CAD build for the part. Positions are in the model's coordinates, mm. A direction names the side the tool comes from. Round coordinates to 2 decimals unless told otherwise and drop trailing zeros. Loops run counter-clockwise (first coordinate to the right, second up) from the corner with the lowest first, then second, coordinate; pieces in that order, holes last. Notation, with made-up numbers: M -0.75,54 L 43.25,54 A19 cw 43.25,87 Z; hole C 35,21.25 d11. An arc over 180 degrees is marked long. Use a Markdown table: item, result. Add a question column.
(1) Band-saw the part on B-B, the plane y = 12. Write the cut outline in (x, z).
(2) Which spindle directions (+Z, -Z, +X, -X, +Y, -Y) get a long thin tool onto all of the face, cutting with end or side? Do faces 4 (the face through (124.456, 4, 13)), 5 (the face through (-81, 27, 25.4)). Say none if no direction does.
(3) Flat gauge pins, fed straight in: P1, Ø2, axis at x = 95.5, y = -0.5, coming from the +Z side; P2, Ø1, axis at x = -89.5, z = 43.5, coming from the +Y side; P3, Ø8, axis at y = 27.5, z = 36.5, coming from the -X side. Where does each tip first touch, or does it go through?
(4) Wall check: L1, parallel to Z at x = 68, y = -40.5; L2, parallel to X at y = 32, z = 48; L3, parallel to X at y = 18.5, z = 28.5. Give the ranges that are in metal, low to high.
(5) Band-saw the part on C-C, the plane z = 33.5. Write the cut outline in (x, y), and give its area (3 significant figures).
(6) Band-saw the part on A-A, the plane x = -75.5. Write the cut outline in (y, z).
(7) Band-saw the part on D-D, the plane x = -49. Write the cut outline in (y, z).
(8) Two-plate mould, pull along X, no slides. Class faces 1 (the face through (-1, -47.706, 13)), 2 (the face through (-78.75, 25.12, 12.52)), 3 (the face through (-70.36, 22.52, 37.92)): released by +X, released by -X, zero draft, split by the parting line, or undercut.
from build123d import *

# Parameters (mm, degrees)
F0_W     = 246.912122
F0_H     = 104.684964
F1_DEPTH = 25.4
F3_D     = 6.35
F2_R     = 11.813862
F4_DEPTH = 25.4


with BuildPart() as f1:
    # F0 (on Top) → F1 (new body)
    with BuildSketch(Plane.XY):
        with Locations((0.999786, 4.636642)):
            Rectangle(F0_W, F0_H)
    extrude(amount=F1_DEPTH)

    # F3 (through all)
    with Locations(Plane.XY.offset(25.4)):
        with Locations((-81.271335, 27.049223)):
            Hole(F3_D / 2)

    # F2 (on face) → F4 (join)
    with BuildSketch(Plane.XY.offset(25.4)):
        with Locations((-81.271335, 27.049223)):
            Circle(F2_R)
    extrude(amount=F4_DEPTH)


solid = f1.part
Return value:
| question | item | result |
|---|---|---|
| 1 | outline | M -122.46,0 L 124.46,0 L 124.46,25.4 L -122.46,25.4 Z |
| 2 | face 4 | +Z, -Z, +X, +Y, -Y |
| 2 | face 5 | -Z |
| 3 | P1 | z = 25.4 |
| 3 | P2 | y = 35.98 |
| 3 | P3 | x = -93.09 |
| 4 | L1 | 0 to 25.4 |
| 4 | L2 | -92 to -70.54 |
| 4 | L3 | -89.42 to -73.12 |
| 5 | outline | C -81.27,27.05 d23.63 |
| 5 | area | 438 mm^2 |
| 6 | outline | M -47.71,0 L 56.98,0 L 56.98,25.4 L 37.36,25.4 L 37.36,50.8 L 16.74,50.8 L 16.74,25.4 L -47.71,25.4 Z |
| 7 | outline | M -47.71,0 L 56.98,0 L 56.98,25.4 L -47.71,25.4 Z |
| 8 | face 1 | zero draft |
| 8 | face 2 | undercut |
| 8 | face 3 | split by the parting line |
